from build123d import *

# Parameters (mm, degrees)
SKETCH1_R                       = 252.5
SKETCH1_R_2                     = 248.75
BOSS_EXTRUDE1_DEPTH             = 21.8
SKETCH2_R                       = 253.75
SKETCH2_R_2                     = 250.5
BOSS_EXTRUDE2_DEPTH             = 1
BOSS_EXTRUDE2_DIRECTION_2_REACH = 359.754


with BuildPart() as part:
    # Sketch1 → Boss-Extrude1 (new body)
    with BuildSketch(Plane.XY):
        Circle(SKETCH1_R)
        Circle(SKETCH1_R_2, mode=Mode.SUBTRACT)
    extrude(amount=BOSS_EXTRUDE1_DEPTH)

    # Sketch2 → Boss-Extrude2 (add)
    with BuildSketch(Plane(origin=(0, 0, 0), x_dir=(-1, 0, 0), z_dir=(0, 0, -1))):
        Circle(SKETCH2_R)
        Circle(SKETCH2_R_2, mode=Mode.SUBTRACT)
    extrude(amount=BOSS_EXTRUDE2_DEPTH)

    # Boss-Extrude2 direction 2: up to this face of the body (flat: up to its plane)
    boss_extrude2_direction_2_end = Plane(part.part.faces().sort_by_distance((-251.785822151, 0, 21.8))[0])
    # Sketch2 → Boss-Extrude2 direction 2 (add, up to the picked face)
    with BuildSketch(Plane(origin=(0, 0, 0), x_dir=(-1, 0, 0), z_dir=(0, 0, -1)), mode=Mode.PRIVATE) as boss_extrude2_direction_2_sk1:
        Circle(SKETCH2_R)
        Circle(SKETCH2_R_2, mode=Mode.SUBTRACT)
    boss_extrude2_direction_2_tool1 = split(extrude(boss_extrude2_direction_2_sk1.sketch, amount=-BOSS_EXTRUDE2_DIRECTION_2_REACH, mode=Mode.PRIVATE), bisect_by=boss_extrude2_direction_2_end, keep=Keep.BOTH, mode=Mode.PRIVATE)
    add(boss_extrude2_direction_2_tool1.solids().sort_by(Axis((253.032287, 0, 0), (0, 0, 1)))[0])

    # SurfaceCut1
    split(bisect_by=Plane(origin=(0, 0, 0), x_dir=(1, 0, 0), z_dir=(0, 1, 0)), keep=Keep.TOP)

    # SurfaceCut2
    split(bisect_by=Plane(origin=(0, 0, 0), x_dir=(0, 0, -1), z_dir=(1, 0, 0)), keep=Keep.TOP)


solid = part.part
Work out the finished part from the listing and answer in its coordinate system (mm). A direction names the side the tool comes from. Coordinates: 2 decimals unless noted, no trailing zeros. Write each loop counter-clockwise with the first axis right and the second up, starting at its lowest first coordinate (ties: lowest second). Pieces come first, ordered by that corner, then holes. Notation, with made-up numbers: M 63,69.5 L 99,69.5 A20 cw 99,78.5 Z; hole C -34,-28.5 d9. An arc over 180 degrees is marked long. Write item = value, one per line.
1. Flat-ended cylindrical pins translate along their axes: pin 1 (1.5 mm diameter, centred on y = 225.5, z = 9.5, fed in from +X); pin 2 (1 mm diameter, centred on y = 28.5, z = 9.5, fed in from -X); pin 3 (3 mm diameter, centred on x = 117.5, z = 9.5, fed in from -Y). Find the tip coordinate at first contact, or state that the pin passes through.
Solution:
pin_1 = 117.8
pin_2 = 247.05
pin_3 = 218.44
2. For faces 1 (the face through (175.17, 179.07, -0.49)), 2 (the face through (177.445, 181.39, 10.24)), determine the directions among +Z, -Z, +X, -X, +Y, -Y from which every point of the face is accessible in a straight line to the end or side of a thin tool.
Solution:
face_1 = -Z, -X, -Y
face_2 = +Z, -Z, +X, +Y
3. The part is cut by section A-A (z = 9). Determine the outline of the cut face in (x, y), then the cut area to 3 significant figures.
Solution:
outline = M 0,248.75 A248.75 cw 248.75,0 L 253.75,0 A253.75 ccw 0,253.75 Z
area = 1,970 mm2
4. Straight lines are drawn through the part: line 1 (Y direction, x = 42, z = 8.75); line 2 (X direction, y = 146.5, z = 6.5); line 3 (Y direction, x = 187, z = 2.25). For each, find the intervals that lie inside material, in ascending order. Write a range as from..to.
Solution:
line_1 = 245.18..250.25
line_2 = 201.03..207.19
line_3 = 164.04..171.52
5. The part is cut by section B-B (x = 60). Determine the outline of the cut face in (y, z).
Solution:
outline = M 241.41,0 L 243.21,0 L 243.21,-1 L 246.55,-1 L 246.55,21.8 L 241.41,21.8 Z
